For this review, take the finished solid that the model builds, in its own axes (mm). Coordinates: 2 decimals unless noted, no trailing zeros. Order: outer loops, then holes, each group sorted by start corner. A loop starts at its lowest first (then second) coordinate and runs counter-clockwise, first axis right, second up. Notation, with made-up numbers: (57, 45) -> (113, 45) arc R30 cw to (113, 74) -> close; hole circle Ø4 at (-38.75, 52.25). An arc over 180 degrees is marked (long way). Write item = value, one per line. Start each with the question number.
1) Consider section B-B on x = 0. Give the boundary of the cut face in (y, z).
2) Insertion check: pin 1 Ø1.2 at (x, y) = (-5, 7.5) entering from -Z. The pin has a flat end and moves straight along its axis. Give the tip position at first contact, or say it passes through.
3) Wall thickness on probe 1 along Y at (x, z) = (0, 0.75); probe 2 along X at (y, z) = (7, 0.6); probe 3 along Y at (x, z) = (8, 0.4): over which ranges is each line inside the solid? List them lowest first. Write a range as [from, to].
4) Consider section A-A on y = 7.5. Give the boundary of the cut face in (x, z), and give its area (3 significant figures).
5) Consider section D-D on x = 10.5. Give the boundary of the cut face in (y, z).
6) Consider section C-C on z = 0.45. Give the boundary of the cut face in (x, y).
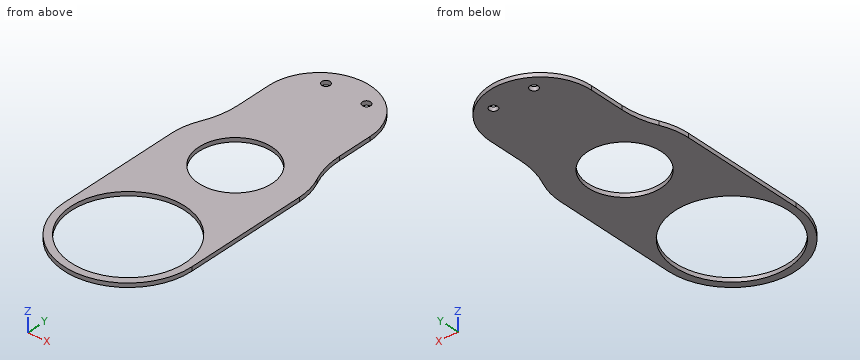
Autodesk Inventor part; units mm, degrees
ref_plane "YZ Plane" through (0, 0, 0) normal (1, 0, 0) x (0, 1, 0)
ref_plane "XZ Plane" through (0, 0, 0) normal (0, 1, 0) x (-1, 0, 0)
ref_plane "XY Plane" through (0, 0, 0) normal (0, 0, 1) x (1, 0, 0)
sketch "スケッチ1" plane through (0, 0, 0) normal (0, 0, 1) x (1, 0, 0)
  circle A0 centre (0, 0) radius 12.5
  circle A1 centre (0, -23.5) radius 15.75
  line L0 (-12.5, 0) -> (-12.5, -13.9181)
  line L1 (12.5, 0) -> (12.5, -13.9181)
  line L2 (0, 0) -> (0, -50.4255)
  point P0 (-15.75, -23.4978)
  point P1 (0.01, 12.5)
  dimension "d0" = 25
  dimension "d1" = 31.5
  dimension "d2" = 23.5
  dimension "d49" = 0
  dimension "d50" = 0
extrude "押し出し2" add sketch "スケッチ1" along normal blind 1
sketch "スケッチ4" plane through (0, 0, 0) normal (0, 0, -1) x (-1, 0, 0)
  arc A0 (12.5, 0) -> (-12.5, 0) centre (0, 0) ccw
  point P0 (-5, 7.5)
  point P1 (5, 7.5)
  dimension "d29" = 10
  dimension "d30" = 5
  dimension "d31" = 7.5
  dimension "d32" = 7.5
hole "Hole3" at (5, 7.5, 0) at (-5, 7.5, 0) direction (0, 0, 1) diameter 2 depth 8 tip angle 118
sketch "スケッチ5" plane through (0, 0, 0) normal (0, 0, -1) x (-1, 0, 0)
  arc A0 (-12.5, -13.9181) -> (12.5, -13.9181) centre (0, -23.5) ccw
hole "Hole4" at (0, -23.5, 0) direction (0, 0, 1) diameter 18 end through all
sketch "スケッチ6" plane through (0, 0, 0) normal (0, 0, -1) x (-1, 0, 0)
  circle A0 centre (0, -23.5) radius 9
  arc A1 (-12.5, -13.9181) -> (12.5, -13.9181) centre (0, -23.5) ccw
  line L0 (12.5, 0) -> (12.5, -13.9181)
  circle A2 centre (0, -53.5) radius 14
  circle A3 centre (0, -53.5) radius 15.75
  line L1 (-15.75, -23.5) -> (-15.75, -53.5)
  line L2 (15.75, -23.5) -> (15.75, -53.5)
  dimension "d51" = 28
  dimension "d52" = 30
  dimension "d53" = 31.5
extrude "押し出し3" add sketch "スケッチ6" against normal blind 1 contours A1 A3 L1 | A1 A3 | A1 L2 A3 picked at (15.0141, -54.7564)
fillet "フィレット2" radius 20 2 edges at (12.5, -13.9181, 0.5) (-12.5, -13.9181, 0.5)
properties part number "JointC3'cover2_2nd" material "アルミニウム 6061"
Answer sheet:
q1.outline = (-69.25, 0) -> (-67.5, 0) -> (-67.5, 1) -> (-69.25, 1) -> close; (-39.5, 0) -> (-32.5, 0) -> (-32.5, 1) -> (-39.5, 1) -> close; (-14.5, 0) -> (12.5, 0) -> (12.5, 1) -> (-14.5, 1) -> close
q2.pin_1 = through
q3.probe_1 = [-69.25, -67.5], [-39.5, -32.5], [-14.5, 12.5]
q3.probe_2 = [-10.36, -5.87], [-4.13, 4.13], [5.87, 10.36]
q3.probe_3 = [-67.07, -64.99], [-42.01, -27.62], [-19.38, 9.6]
q4.outline = (-10, 0) -> (-6, 0) -> (-6, 1) -> (-10, 1) -> close; (-4, 0) -> (4, 0) -> (4, 1) -> (-4, 1) -> close; (6, 0) -> (10, 0) -> (10, 1) -> (6, 1) -> close
q4.area = 16.0 mm2
q5.outline = (-65.24, 0) -> (-62.76, 0) -> (-62.76, 1) -> (-65.24, 1) -> close; (-44.24, 0) -> (6.78, 0) -> (6.78, 1) -> (-44.24, 1) -> close
q6.outline = (-15.75, -53.5) arc R15.75 ccw to (15.75, -53.5) -> (15.75, -23.5) arc R15.75 ccw to (14.32, -16.94) arc R20 cw to (12.5, -8.61) -> (12.5, 0) arc R12.5 ccw to (-12.5, 0) -> (-12.5, -8.61) arc R20 cw to (-14.32, -16.94) arc R15.75 ccw to (-15.75, -23.5) -> close; hole circle Ø28 at (0, -53.5); hole circle Ø18 at (0, -23.5); hole circle Ø2 at (-5, 7.5); hole circle Ø2 at (5, 7.5)
